Read the model definition and answer for the solid it produces. Units are mm, in the model's axes. Face numbers are marked on the shaded views. A direction names the side the tool comes from. Round coordinates to 2 decimals unless told otherwise and drop trailing zeros. Order: outer loops, then holes, each group sorted by start corner. A loop starts at its lowest first (then second) coordinate and runs counter-clockwise, first axis right, second up. Notation, with made-up numbers: (78.5, 68) -> (83.5, 68) arc R7 cw to (83.5, 75) -> close; hole circle Ø4 at (58, 2). An arc over 180 degrees is marked (long way). Answer as a JSON object with one key per item and string values. Group by question number.
Item 1: Section D-D, the plane y = 10.5 is taken. Write down the section's boundary in (x, z), plus the area to 3 significant figures.
Item 2: Section B-B, the plane x = -9.5 is taken. Write down the section's boundary in (y, z).
Item 3: For the marked faces 1, 2 and 3, determine the directions among +Z, -Z, +X, -X, +Y, -Y from which every point of the face is accessible in a straight line to the end or side of a thin tool.
Item 4: Given P1, Ø15.5, axis at x = 7.5, y = 10, coming from the -Z side; P2, Ø2, axis at y = -8, z = 24.5, coming from the +X side; P3, Ø3, axis at x = 3, y = -3, coming from the +Z side, each flat-ended and moving along its own axis, determine where each tip first touches the part or whether it passes through.
Item 5: Section A-A, the plane y = -14 is taken. Write down the section's boundary in (x, z), plus the area to 3 significant figures.
Item 6: Consider probe 1 along X at (y, z) = (28.5, 18); probe 2 along Z at (x, y) = (-41.5, -22.5); probe 3 along Z at (x, y) = (-32, -18). Determine where each line is inside the solid, lowest interval first. Write a range as from..to.
Item 7: Section C-C, the plane z = 4.5 is taken. Write down the section's boundary in (x, y) (3 decimals), plus the area to 3 significant figures.
Item 8: The mould has two halves that part along Y. Classify the marked faces 4, 5, 6 and 7: pulls with the +Y half, pulls with the -Y half, needs draft (parallel to the pull), parting line crosses it, or undercut.
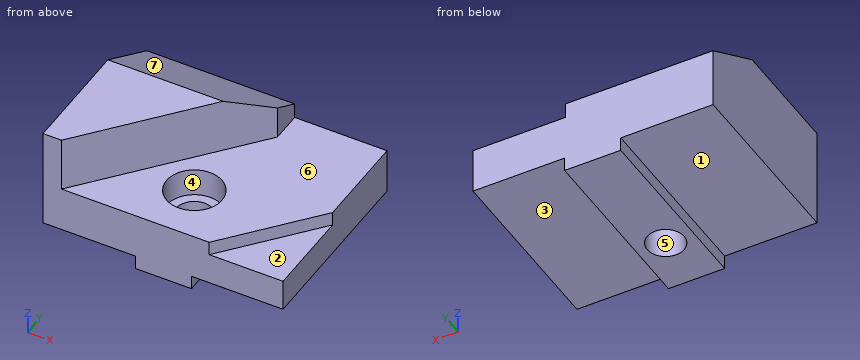
from build123d import *

# Parameters (mm, degrees)
F1_DEPTH       = 31.75
F3_DEPTH       = 19.05
F5_DEPTH       = 4.826
F7_DEPTH       = 52.4256
F9_D           = 12.7
F9_CBORE_D     = 19.05
F9_CBORE_DEPTH = 9.652


with BuildPart() as f1:
    # F0 (on Front) → F1 (new body, symmetric)
    with BuildSketch(Plane.XZ):
        Polygon((-22.139631, -8.012854), (-2.835631, -8.012854), (-2.835631, -3.186854), (28.660369, -3.186854), (28.660369, 12.561146), (-3.089631, 12.561146), (-3.089631, 31.611146), (-53.889631, 31.611146), (-53.889631, -3.186854), (-22.139631, -3.186854), align=None)
    extrude(amount=F1_DEPTH, both=True)

    # F2 (on face) → F3 (cut)
    with BuildSketch(Plane.XY.offset(31.611146)):
        Polygon((-3.089631, 21.223447), (-47.539631, -31.75), (-3.089631, -31.75), align=None)
    extrude(amount=-F3_DEPTH, mode=Mode.SUBTRACT)

    # F4 (on face) → F5 (cut)
    with BuildSketch(Plane.XY.offset(12.561146)):
        Polygon((3.260369, -31.75), (28.660369, -31.75), (28.660369, -1.479459), align=None)
    extrude(amount=-F5_DEPTH, mode=Mode.SUBTRACT)

    # F6 (on face) → F7 (cut)
    with BuildSketch(Plane(origin=(-53.889631, 0, 0), x_dir=(0, -1, 0), z_dir=(-1, 0, 0))):
        Polygon((-31.75, 17.826331), (-7.874, 31.611146), (-31.75, 31.611146), align=None)
    extrude(amount=-F7_DEPTH, mode=Mode.SUBTRACT)

    # F9 (through all)
    with Locations(Plane.XY.offset(12.561146)):
        with Locations((-12.574879, -12.7)):
            CounterBoreHole(F9_D / 2, F9_CBORE_D / 2, F9_CBORE_DEPTH)


solid = f1.part
Values found:
{
 "1": {"outline": "(-53.89, -3.19) -> (-22.14, -3.19) -> (-22.14, -8.01) -> (-2.84, -8.01) -> (-2.84, -3.19) -> (28.66, -3.19) -> (28.66, 12.56) -> (-12.09, 12.56) -> (-12.09, 30.1) -> (-53.89, 30.1) -> close", "area": "2,130 mm2"},
 "2": {"outline": "(-31.75, -8.01) -> (-18.26, -8.01) -> (-18.26, 2.91) -> (-21.72, 2.91) -> (-21.72, 12.56) -> (-31.75, 12.56) -> close; (-7.14, -8.01) -> (31.75, -8.01) -> (31.75, 17.83) -> (13.58, 28.31) -> (13.58, 12.56) -> (-3.68, 12.56) -> (-3.68, 2.91) -> (-7.14, 2.91) -> close"},
 "3": {"face 1": "-Z, -X, +Y, -Y", "face 2": "+Z, +X, -Y", "face 3": "-Z, +X, +Y, -Y"},
 "4": {"P1": "z = -3.19", "P2": "x = -26.77", "P3": "z = 12.56"},
 "5": {"outline": "(-53.89, -3.19) -> (-22.14, -3.19) -> (-22.14, -8.01) -> (-18.79, -8.01) -> (-18.79, 2.91) -> (-22.01, 2.91) -> (-22.01, 12.56) -> (-32.65, 12.56) -> (-32.65, 31.61) -> (-53.89, 31.61) -> close; (-6.36, -8.01) -> (-2.84, -8.01) -> (-2.84, -3.19) -> (28.66, -3.19) -> (28.66, 7.74) -> (18.15, 7.74) -> (18.15, 12.56) -> (-3.14, 12.56) -> (-3.14, 2.91) -> (-6.36, 2.91) -> close", "area": "1,430 mm2"},
 "6": {"probe 1": "-53.89..-3.09", "probe 2": "-3.19..31.61", "probe 3": "-3.19..12.56"},
 "7": {"outline": "(-53.89, -31.75) -> (28.66, -31.75) -> (28.66, 31.75) -> (-53.89, 31.75) -> close; hole circle Ø19.05 at (-12.575, -12.7)", "area": "4,960 mm2"},
 "8": {"face 4": "undercut", "face 5": "undercut", "face 6": "needs draft", "face 7": "pulls with the +Y half"}
}
